The model under review builds one solid part; all positions refer to its coordinate system, in mm. Coordinates: 2 decimals unless noted, no trailing zeros. Write each loop counter-clockwise with the first axis right and the second up, starting at its lowest first coordinate (ties: lowest second). Pieces come first, ordered by that corner, then holes. Notation, with made-up numbers: (24.5, 88.5) - (65.5, 88.5) arc R21 ccw to (65.5, 106.5) - close; hole circle Ø8 at (43, -10). An arc over 180 degrees is marked (long way). Put each result on its own line as item: value.
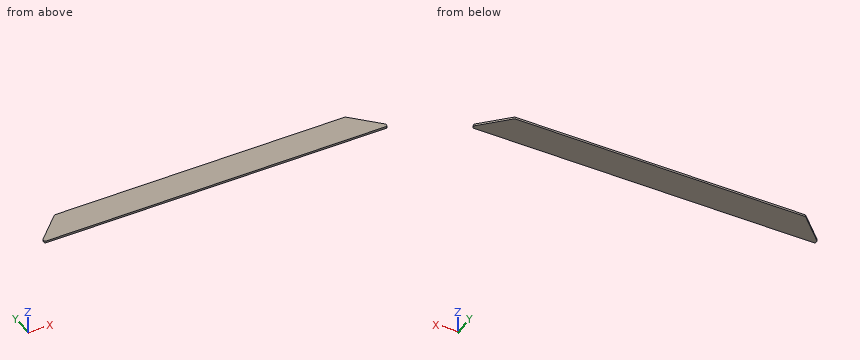
from build123d import *

# Parameters (mm, degrees)
BOSS_EXTRUDE1_DEPTH = 1.6
FILLET1_R           = 1
BOSS_EXTRUDE2_DEPTH = 1.6


with BuildPart() as part:
    # Sketch1 → Boss-Extrude1 (new body)
    with BuildSketch(Plane.XY):
        with BuildLine():
            Line((21.213203436, 24), (0, 2.786796564))
            Line((0, 2.786796564), (0, 0))
            Line((0, 0), (42, 0))
            Line((42, 0), (42, 11))
            ThreePointArc((42, 11), (43.171572875, 13.828427125), (46, 15))
            Line((46, 15), (234, 15))
            ThreePointArc((234, 15), (236.828427125, 13.828427125), (238, 11))
            Line((238, 11), (238, 0))
            Line((238, 0), (280, 0))
            Line((280, 0), (280, 2.786796564))
            Line((280, 2.786796564), (258.786796564, 24))
            Line((258.786796564, 24), (21.213203436, 24))
        make_face()
    extrude(amount=BOSS_EXTRUDE1_DEPTH)

    # Fillet1
    fillet1_edges = [part.edges().sort_by_distance(p)[0] for p in [
        (0, 0, 0.8),
        (0, 2.786796564, 0.8),
        (21.213203436, 24, 0.8),
        (258.786796564, 24, 0.8),
        (280, 2.786796564, 0.8),
        (280, 0, 0.8),
    ]]
    fillet(fillet1_edges, radius=FILLET1_R)

    # Sketch1<3> → Boss-Extrude2 (add)
    with BuildSketch(Plane.XY):
        with BuildLine():
            Line((42, 11), (42, 0))
            Line((42, 0), (238, 0))
            Line((238, 0), (238, 11))
            ThreePointArc((238, 11), (236.828427125, 13.828427125), (234, 15))
            Line((234, 15), (46, 15))
            ThreePointArc((46, 15), (43.171572875, 13.828427125), (42, 11))
        make_face()
    extrude(amount=BOSS_EXTRUDE2_DEPTH)


solid = part.part
1. Consider section A-A on z = 0.25. State the section outline as (x, y) points.
Determined:
outline: (0, 1) arc R1 ccw to (1, 0) - (279, 0) arc R1 ccw to (280, 1) - (280, 2.37) arc R1 ccw to (279.71, 3.08) - (259.08, 23.71) arc R1 ccw to (258.37, 24) - (21.63, 24) arc R1 ccw to (20.92, 23.71) - (0.29, 3.08) arc R1 ccw to (0, 2.37) - close
2. Consider section B-B on y = 8.75. State the section outline as (x, z) points, plus the area to 3 significant figures.
Determined:
outline: (5.96, 0) - (274.04, 0) - (274.04, 1.6) - (5.96, 1.6) - close
area: 429 mm^2
3. Consider section C-C on y = 19.25. State the section outline as (x, z) points.
Determined:
outline: (16.46, 0) - (263.54, 0) - (263.54, 1.6) - (16.46, 1.6) - close
4. To check wall thickness, follow probe 1 along X at (y, z) = (13.5, 0.45); probe 2 along X at (y, z) = (9.5, 1.35); probe 3 along Y at (x, z) = (264.5, 0.4). State the ranges of each line that lie inside material, in increasing order.
Determined:
probe 1: x = 10.71 to 269.29
probe 2: x = 6.71 to 273.29
probe 3: y = 0 to 18.29
